Autodesk Inventor part; units mm, degrees
ref_plane "YZ Plane" through (0, 0, 0) normal (1, 0, 0) x (0, 1, 0)
ref_plane "XZ Plane" through (0, 0, 0) normal (0, 1, 0) x (-1, 0, 0)
ref_plane "XY Plane" through (0, 0, 0) normal (0, 0, 1) x (1, 0, 0)
sketch "Sketch1" plane through (0, 0, 0) normal (0, 0, 1) x (1, 0, 0)
  line L0 (8.8, 13.8) -> (-8.8, 13.8)
  line L1 (-8.8, 13.8) -> (-8.8, -13.8)
  line L2 (-8.8, -13.8) -> (8.8, -13.8)
  line L3 (8.8, -13.8) -> (8.8, 13.8)
  line L4 (8.8, 13.8) -> (-8.8, -13.8) construction
  line L5 (-8.8, 13.8) -> (8.8, -13.8) construction
  line L6 (8.8, 0) -> (-8.8, 0) construction
  line L7 (2.5, -13.8) -> (-2.5, -13.8)
  line L8 (-2.5, -8.8) -> (2.5, -8.8)
  line L9 (2.5, -8.8) -> (2.5, -13.8)
  line L10 (2.5, -13.8) -> (-2.5, -8.8) construction
  line L11 (-2.5, -13.8) -> (2.5, -8.8) construction
  line L12 (-2.5, -8.8) -> (-2.5, -13.8)
  line L13 (3.8, -2.5) -> (8.8, -2.5)
  line L14 (3.8, 8.8) -> (-3.8, 8.8)
  line L15 (-3.8, 8.8) -> (-3.8, -8.8)
  line L16 (-3.8, -8.8) -> (3.8, -8.8)
  line L17 (3.8, -8.8) -> (3.8, 8.8)
  line L18 (3.8, 8.8) -> (-3.8, -8.8) construction
  line L19 (-3.8, 8.8) -> (3.8, -8.8) construction
  line L20 (-3.8, -2.5) -> (-8.8, -2.5)
  line L21 (2.5, 13.8) -> (-2.5, 13.8)
  line L22 (-2.5, 8.8) -> (2.5, 8.8)
  line L23 (2.5, 8.8) -> (2.5, 13.8)
  line L24 (2.5, 13.8) -> (-2.5, 8.8) construction
  line L25 (-2.5, 13.8) -> (2.5, 8.8) construction
  line L26 (-2.5, 8.8) -> (-2.5, 13.8)
  line L27 (3.8, 2.5) -> (8.8, 2.5)
  line L28 (-3.8, 2.5) -> (-8.8, 2.5)
  point P0 (0, 0)
  dimension "d0" = 17.6
  dimension "d1" = 27.6
  dimension "d5" = 5
  dimension "d7" = 7.6
  dimension "d8" = 17.6
extrude "Extrusion1" add sketch "Sketch1" against normal blind 3 contours L3 L27 L17 L14 L23 L0 | L26 L14 L15 L28 L1 L0 | L3 L2 L9 L16 L17 L13 | L20 L15 L16 L12 L2 L1
sketch "Sketch2" plane through (0, 0, 0) normal (0, 0, 1) x (1, 0, 0)
  line L0 (11, 16) -> (-11, 16)
  line L1 (-11, 16) -> (-11, -16)
  line L2 (-11, -16) -> (11, -16)
  line L3 (11, -16) -> (11, 16)
  line L4 (11, 16) -> (-11, -16) construction
  line L5 (-11, 16) -> (11, -16) construction
  line L6 (11, 16) -> (11.4, 16)
  line L7 (11.4, 16) -> (11.4, -16)
  line L8 (11.4, -16) -> (11, -16)
  line L9 (11, -16) -> (11, 16)
  point P0 (0, 0)
  dimension "d11" = 22
  dimension "d12" = 32
  dimension "d18" = 0.4
extrude "Extrusion2" add sketch "Sketch2" along normal blind 2
sketch "Sketch3" plane through (11.4, -16, 0) normal (1, 0, 0) x (0, 0, -1)
  line L0 (-2, 32) -> (-2, 0)
  line L1 (-2, 0) -> (58, 0)
  line L2 (58, 0) -> (58, 32)
  line L3 (58, 32) -> (-2, 32)
  line L4 (-2, 32) -> (-2, 0)
  point P0 (0, 16)
  dimension "d15" = 60
extrude "Extrusion3" add sketch "Sketch3" along normal blind 2
sketch "Sketch5" plane through (11.4, -16, 0) normal (-1, 0, 0) x (0, 0, 1)
  line L0 (-2, 14.5) -> (0, 14.5)
  line L1 (0, 14.5) -> (0, 17.5)
  line L2 (0, 17.5) -> (-2, 17.5)
  line L3 (-2, 17.5) -> (-2, 14.5)
  point P0 (0, 16)
  point P1 (0, 16)
  dimension "d19" = 2
  dimension "d20" = 3
extrude "Extrusion4" cut sketch "Sketch5" against normal up to surface (2 mm away)
sketch "Sketch6" plane through (13.4, -16, 0) normal (1, 0, 0) x (0, 0, -1)
  line L0 (0, 32) -> (0, 0)
  line L1 (-2, 32) -> (0, 32)
  line L2 (0, 32) -> (0, 0)
  line L3 (0, 0) -> (-2, 0)
  line L4 (-2, 0) -> (-2, 32)
  point P0 (0, 16)
extrude "Extrusion5" add sketch "Sketch6" along normal blind 22
sketch "Sketch7" plane through (13.4, -16, 0) normal (1, 0, 0) x (0, 0, -1)
  line L0 (0, 0) -> (58, 0)
  line L1 (58, 0) -> (58, 32)
  line L2 (58, 32) -> (0, 32)
  line L3 (54.5, 28) -> (5.5, 28) construction
  line L4 (5.5, 28) -> (5.5, 4) construction
  line L5 (5.5, 4) -> (54.5, 4) construction
  line L6 (54.5, 4) -> (54.5, 28) construction
  line L7 (54.5, 28) -> (5.5, 4) construction
  line L8 (5.5, 28) -> (54.5, 4) construction
  circle A0 centre (47, 7.4) radius 2.5
  circle A1 centre (47, 7.4) radius 1.4
  circle A2 centre (13, 24.6) radius 2.5
  circle A3 centre (13, 24.6) radius 1.4
  line L9 (0, 0) -> (58, 0)
  line L10 (58, 0) -> (58, 32)
  line L11 (2, 0) -> (58, 32) construction
  point P0 (30, 16)
  point P1 (30, 16)
  dimension "d37" = 49
  dimension "d38" = 24
  dimension "d39" = 5
  dimension "d40" = 2.8
  dimension "d41" = 5
  dimension "d42" = 2.8
  dimension "d43" = 3.4
  dimension "d44" = 7.5
  dimension "d45" = 3.4
  dimension "d46" = 7.5
extrude "Extrusion6" add sketch "Sketch7" along normal blind 4
properties part number "prototype_5_testPart1_3DPrint"
Can you work these out from the model? Positions are in its coordinate system, mm. A direction names the side the tool comes from. Round coordinates to 2 decimals unless told otherwise and drop trailing zeros. Order: outer loops, then holes, each group sorted by start corner. A loop starts at its lowest first (then second) coordinate and runs counter-clockwise, first axis right, second up. Notation, with made-up numbers: (81, 64) -> (106, 64) arc R17 cw to (106, 93) -> close; hole circle Ø6 at (1, -15.75). An arc over 180 degrees is marked (long way). Return JSON: item names as keys, results as strings. Group by question number.
1. If we section it at D-D, the plane y = -12.5: Write out the boundary of the cut face in (x, z).
2. Which directions (+Z, -Z, +X, -X, +Y, -Y) give clear straight access to the entire face, cutting with the end or side of a thin tool? Please do faces 5 (the face through (-6, -2.5, -1)), 6 (the face through (3, -8.8, -1)), 7 (the face through (15.37, -7.64, -49.31)), 8 (the face through (-6, -8, -3)), 9 (the face through (2.5, -11, -1)).
3. Will these pins go through, and if not, where does the flat tip stop? pin 1 (4 mm diameter, centred on y = 4, z = -37.5, fed in from +X); pin 2 (5 mm diameter, centred on x = 7, z = -21.5, fed in from -Y); pin 3 (3 mm diameter, centred on x = 9, y = -9.5, fed in from -Z); pin 4 (0.6 mm diameter, centred on x = 3.5, z = -1.5, fed in from -Y).
4. I need wall thicknesses on line 1 (Y direction, x = 15.4, z = -47); line 2 (Z direction, x = 14, y = -8); line 3 (Y direction, x = 14.5, z = -13). Which ranges of each line are inside material? Lowest first, please. Write a range as [from, to].
5. If we section it at A-A, the plane z = -13: Write out the boundary of the cut face in (x, y).
6. If we section it at C-C, the plane x = -7: Write out the boundary of the cut face in (y, z).
7. If we section it at B-B, the plane y = 5: Write out the boundary of the cut face in (x, z), then the cut area to 3 significant figures.
8. We'd pull the mould along X, two halves only. Please class faces 1 (the face through (3.8, 6, -1)), 2 (the face through (13.4, 0, -29)), 3 (the face through (-3, 8.8, -1)), 4 (the face through (12, 0, 2)): released by +X, released by -X, zero draft, split by the parting line, or undercut.
Output values:
{
 "1": {"outline": "(-11, 0) -> (-8.8, 0) -> (-8.8, -3) -> (-2.5, -3) -> (-2.5, 0) -> (2.5, 0) -> (2.5, -3) -> (8.8, -3) -> (8.8, 0) -> (11.4, 0) -> (11.4, -58) -> (13.4, -58) -> (13.4, 0) -> (35.4, 0) -> (35.4, 2) -> (-11, 2) -> close"},
 "2": {"face 5": "-Z, -X", "face 6": "-Z", "face 7": "+X", "face 8": "-Z, -X, +Y, -Y", "face 9": "-Z, +Y, -Y"},
 "3": {"pin 1": "x = 13.4", "pin 2": "through", "pin 3": "z = -3", "pin 4": "y = -13.8"},
 "4": {"line 1": "[-11.1, -10], [-7.2, -6.1]", "line 2": "[-49.43, -48.26], [-45.74, -44.57], [0, 2]", "line 3": "[6.1, 7.2], [10, 11.1]"},
 "5": {"outline": "(11.4, -16) -> (13.4, -16) -> (13.4, 6.1) -> (17.4, 6.1) -> (17.4, 7.2) -> (13.4, 7.2) -> (13.4, 10) -> (17.4, 10) -> (17.4, 11.1) -> (13.4, 11.1) -> (13.4, 16) -> (11.4, 16) -> close"},
 "6": {"outline": "(-16, 0) -> (-13.8, 0) -> (-13.8, -3) -> (-2.5, -3) -> (-2.5, 0) -> (2.5, 0) -> (2.5, -3) -> (13.8, -3) -> (13.8, 0) -> (16, 0) -> (16, 2) -> (-16, 2) -> close"},
 "7": {"outline": "(-11, 0) -> (-8.8, 0) -> (-8.8, -3) -> (-3.8, -3) -> (-3.8, 0) -> (3.8, 0) -> (3.8, -3) -> (8.8, -3) -> (8.8, 0) -> (11.4, 0) -> (11.4, -58) -> (13.4, -58) -> (13.4, 0) -> (35.4, 0) -> (35.4, 2) -> (-11, 2) -> close", "area": "239 mm²"},
 "8": {"face 1": "undercut", "face 2": "released by +X", "face 3": "undercut", "face 4": "zero draft"}
}
